from build123d import *

# Parameters (mm, degrees)
SKETCH1_R           = 4.4
BOSS_EXTRUDE1_DEPTH = 15


with BuildPart() as part:
    # Sketch1 → Boss-Extrude1 (new body)
    with BuildSketch(Plane(origin=(0, 0, 0), x_dir=(1, 0, 0), z_dir=(0, 1, 0))):
        with BuildLine():
            Line((0, 5), (0, 4.912292599))
            Line((0, 4.912292599), (0.042868928, 4.912292599))
            Line((0.042868928, 4.912292599), (0.043632677, 4.999809615))
            ThreePointArc((0.043632677, 4.999809615), (3.550926878, 3.520073622), (5, 0))
            Line((5, 0), (4.915051898, 0))
            Line((4.915051898, 0), (4.915051898, -0.042893008))
            Line((4.915051898, -0.042893008), (4.999809615, -0.043632677))
            ThreePointArc((4.999809615, -0.043632677), (3.535533906, -3.535533906), (0.043632677, -4.999809615))
            Line((0.043632677, -4.999809615), (0.042868928, -4.912292599))
            Line((0.042868928, -4.912292599), (0, -4.912292599))
            Line((0, -4.912292599), (0, -5))
            ThreePointArc((0, -5), (-3.520073622, -3.550926878), (-4.999809615, -0.043632677))
            Line((-4.999809615, -0.043632677), (-4.915051898, -0.042893008))
            Line((-4.915051898, -0.042893008), (-4.915051898, 0))
            Line((-4.915051898, 0), (-5, 0))
            ThreePointArc((-5, 0), (-3.535533906, 3.535533906), (0, 5))
        make_face()
        with Locations(Location((0, 0, 0), (0, 0, 270))):
            Circle(SKETCH1_R, mode=Mode.SUBTRACT)
    extrude(amount=BOSS_EXTRUDE1_DEPTH)


solid = part.part
Could you check a few things on this model? Use its own coordinates, in mm. Give positions to 0.01 mm unless a question says otherwise; leave off trailing zeros. Order: outer loops, then holes, each group sorted by start corner. A loop starts at its lowest first (then second) coordinate and runs counter-clockwise, first axis right, second up. Notation, with made-up numbers: (42, 68.5) -> (66, 68.5) arc R7 ccw to (66, 75.5) -> close; hole circle Ø1 at (-13, 47.25). An arc over 180 degrees is marked (long way). Return JSON: item names as keys, results as strings.
1. Imagine slicing it at A-A on y = 2.75. List the corners of the cut face in (x, z) for me.
Answer list:
{"outline": "(-5, 0) arc R5 ccw to (0, -5) -> (0, -4.91) -> (0.04, -4.91) -> (0.04, -5) arc R5 ccw to (5, 0) -> (4.92, 0) -> (4.92, 0.04) -> (5, 0.04) arc R5 ccw to (0.04, 5) -> (0.04, 4.91) -> (0, 4.91) -> (0, 5) arc R5 ccw to (-5, 0.04) -> (-4.92, 0.04) -> (-4.92, 0) -> close; hole circle Ø8.8 at (0, 0)"}
2. For pin 1 Ø2 at (x, y) = (2.5, 12.5) entering from +Z; pin 2 Ø3 at (x, y) = (2, 12) entering from -Z; pin 3 Ø4 at (x, y) = (-2.5, 13.5) entering from +Z, each with a flat end and sliding along its axis, tell me the tip position at first contact or that it passes through.
Answer list:
{"pin 1": "stops at z = 4.77", "pin 2": "stops at z = -4.97", "pin 3": "stops at z = 4.97"}
3. Thinking about a two-plate mould opening in Z: for faces 1 (the cylindrical face through (3.51, 7.4, -3.56)), 2 (the cylindrical face through (-3, 7, 4)), 3 (the cylindrical face through (4.363, 7.395, -0.573)), which applies, pulls with the +Z half, pulls with the -Z half, needs draft (parallel to the pull), parting line crosses it, or undercut?
Answer list:
{"face 1": "pulls with the -Z half", "face 2": "pulls with the +Z half", "face 3": "undercut"}
4. I need wall thicknesses on line 1 (X direction, y = 12.5, z = -1.25); line 2 (Z direction, x = 0.5, y = 2.75); line 3 (X direction, y = 1.5, z = 3.5). Which ranges of each line are inside material? Lowest first, please. Write a range as from..to.
Answer list:
{"line 1": "x = -4.84..-4.22, 4.22..4.84", "line 2": "z = -4.97..-4.37, 4.37..4.97", "line 3": "x = -3.57..-2.67, 2.67..3.57"}
5. Imagine slicing it at C-C on x = -3.75. List the corners of the cut face in (y, z) for me, then the cut area to 3 significant figures.
Answer list:
{"outline": "(0, -3.31) -> (15, -3.31) -> (15, -2.3) -> (0, -2.3) -> close; (0, 2.3) -> (15, 2.3) -> (15, 3.31) -> (0, 3.31) -> close", "area": "30.2 mm2"}
6. Imagine slicing it at B-B on z = -1.5. List the corners of the cut face in (x, y) for me.
Answer list:
{"outline": "(-4.77, 0) -> (-4.14, 0) -> (-4.14, 15) -> (-4.77, 15) -> close; (4.14, 0) -> (4.77, 0) -> (4.77, 15) -> (4.14, 15) -> close"}
